Autodesk Fusion 360 part; units mm, degrees
sketch "Skizze1" plane through (0, 0, 0) normal (0, 1, 0) x (1, 0, 0)
  line L0 (-7.3758, -5.9007) -> (-2.3758, -5.9007)
  line L1 (-2.3758, -5.9007) -> (-2.3758, -0.9007)
  line L2 (-2.3758, -0.9007) -> (-7.3758, -0.9007)
  line L3 (-7.3758, -0.9007) -> (-7.3758, -5.9007)
  circle A0 centre (-5.9, -4.4) radius 1.35
  dimension "d1" = 5
  dimension "d2" = 5
  dimension "d8" = 2.7
extrude "Extrusion1" add sketch "Skizze1" along normal blind 3 contours L0 L1 L2 L3 | A0
sketch "Skizze3" plane through (0, 0, 0) normal (0, -1, 0) x (1, 0, 0)
  line L0 (-7.3758, 5.9007) -> (-7.3758, 0.9007)
  line L1 (-7.3758, 0.9007) -> (-2.3758, 0.9007)
  line L2 (-2.3758, 0.9007) -> (-2.3758, 5.9007)
  line L3 (-2.3758, 5.9007) -> (-7.3758, 5.9007)
  circle A0 centre (-5.9, 4.4) radius 1.35
  dimension "d9" = 2.7
extrude "Extrusion3" add sketch "Skizze3" along normal blind 8 contours A0
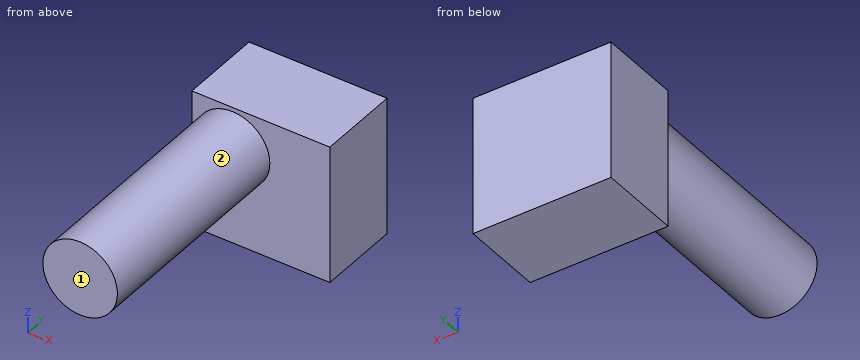
Source: CAD feature listing. Evaluate the final solid. Frame: model axes, mm. Face numbers are marked on the shaded views. A direction names the side the tool comes from. Coordinates: 2 decimals unless noted, no trailing zeros. Order: outer loops, then holes, each group sorted by start corner. A loop starts at its lowest first (then second) coordinate and runs counter-clockwise, first axis right, second up. Notation, with made-up numbers: M 57.25,-22 L 107.25,-22 A35 ccw 107.25,10 Z; hole C 47.25,27.5 d5. An arc over 180 degrees is marked long. Write each question's results on one line, items separated by ' | '. Start each with the question number.
1) Section query B-B (x = -6.75). Return the cut outline in (y, z).
2) Access query for the marked faces 1 and 2. Directions: +Z, -Z, +X, -X, +Y, -Y. A direction counts if a zero-diameter tool reaches every point of the face in a straight line with its end or side. Return the directions, or none.
3) Contact query for flat-ended pins moving along their axis: pin 1 Ø1.5 at (x, z) = (-4, 2.5) entering from -Y; pin 2 Ø3 at (y, z) = (-4.5, 2) entering from -X; pin 3 Ø1 at (y, z) = (-4, 4.5) entering from -X. Output: stop coordinate, or through.
4) Line query: line 1 (Y direction, x = -4.85, z = 2.7); line 2 (Z direction, x = -5.1, y = -0.75); line 3 (Z direction, x = -7, y = -5.25). Output: solid intervals per line, ascending. Write a range as from..to.
5) Section query A-A (z = 4.4). Return the cut outline in (x, y).
6) Section query D-D (x = -2.9). Return the cut outline in (y, z).
7) Section query C-C (y = -4.5). Return the cut outline in (x, z).
Answers:
1) outline: M -8,3.35 L 0,3.35 L 0,0.9 L 3,0.9 L 3,5.9 L 0,5.9 L 0,5.45 L -8,5.45 Z
2) face 1: +Z, -Z, +X, -X, -Y | face 2: -Y
3) pin 1: stops at y = 0 | pin 2: stops at x = -6.91 | pin 3: stops at x = -7.25
4) line 1: y = 0..3 | line 2: z = 3.31..5.49 | line 3: z = 3.62..5.18
5) outline: M -7.38,0 L -7.25,0 L -7.25,-8 L -4.55,-8 L -4.55,0 L -2.38,0 L -2.38,3 L -7.38,3 Z
6) outline: M 0,0.9 L 3,0.9 L 3,5.9 L 0,5.9 Z
7) outline: C -5.9,4.4 d2.7
